Input: part model. Units: mm. Frame: model coordinates. A direction names the side the tool comes from. Round coordinates to 2 decimals unless told otherwise and drop trailing zeros. Loops run counter-clockwise (first coordinate to the right, second up) from the corner with the lowest first, then second, coordinate; pieces in that order, holes last.
1) Draft query along Z for faces 4 (the face through (-16, 2, 32.3)), 5 (the face through (-46, 2, -4)), 6 (the face through (-8, 2, -29)). Return one class per face: pulls with the +Z half, pulls with the -Z half, needs draft (parallel to the pull), parting line crosses it, or undercut.
2) Ray query, line 1 along X through (y, z) = (1.5, -10.5); line 2 along Z through (x, y) = (-41.5, 0.45). Return the intervals inside material, ascending.
3) Access query for faces 1 (the face through (-44, 2, -24)), 2 (the face through (44, 2, 25)), 3 (the face through (28, 2, 31)). Directions: +Z, -Z, +X, -X, +Y, -Y. A direction counts if a zero-diameter tool reaches every point of the face in a straight line with its end or side. Return the directions, or none.
4) First-contact query: pin 1 (1.6 mm diameter, centred on y = 1, z = 9, fed in from -X); pin 2 (1 mm diameter, centred on y = 1, z = -31.5, fed in from -X); pin 3 (1.5 mm diameter, centred on y = 3, z = 22, fed in from +X). Flat tips, straight axial feed; report the tip coordinate or a pass-through.
5) Section A-A, the plane x = -39. Return loops of the section in (y, z), and give its area (3 significant figures).
from build123d import *

# Parameters (mm, degrees)
ESQUISSE4_W                    = 88
ESQUISSE4_H                    = 58
BOSS_EXTRU_3_DEPTH             = 3.3
ESQUISSE5_W                    = 8
ESQUISSE5_H                    = 3.3
BOSS_EXTRU_6_DEPTH             = 3.3
R_P_TITION_LIN_AIRE2_COUNT     = 3
R_P_TITION_LIN_AIRE2_PITCH     = 16
R_P_TITION_LIN_AIRE2_COL_COUNT = 3
R_P_TITION_LIN_AIRE2_COL_PITCH = 16
SYM_TRIE1_COPY_1_SKETCH_W      = 8
SYM_TRIE1_COPY_1_SKETCH_H      = 3.3
SYM_TRIE1_COPY_1_DEPTH         = 3.3
SYM_TRIE1_COPY_2_SKETCH_W      = 8
SYM_TRIE1_COPY_2_SKETCH_H      = 3.3
SYM_TRIE1_COPY_2_DEPTH         = 3.3
SYM_TRIE1_COPY_3_SKETCH_W      = 8
SYM_TRIE1_COPY_3_SKETCH_H      = 3.3
SYM_TRIE1_COPY_3_DEPTH         = 3.3
SYM_TRIE1_COPY_4_SKETCH_W      = 8
SYM_TRIE1_COPY_4_SKETCH_H      = 3.3
SYM_TRIE1_COPY_4_DEPTH         = 3.3
ESQUISSE6_W                    = 3.3
ESQUISSE6_H                    = 8
BOSS_EXTRU_7_DEPTH             = 3.3
R_P_TITION_LIN_AIRE3_COUNT     = 2
R_P_TITION_LIN_AIRE3_PITCH     = 16
R_P_TITION_LIN_AIRE3_COL_COUNT = 2
R_P_TITION_LIN_AIRE3_COL_PITCH = 16
SYM_TRIE2_COPY_1_SKETCH_W      = 3.3
SYM_TRIE2_COPY_1_SKETCH_H      = 8
SYM_TRIE2_COPY_1_DEPTH         = 3.3
SYM_TRIE2_COPY_2_SKETCH_W      = 3.3
SYM_TRIE2_COPY_2_SKETCH_H      = 8
SYM_TRIE2_COPY_2_DEPTH         = 3.3


with BuildPart() as part:
    # Esquisse4 → Boss.-Extru.3 (new body)
    with BuildSketch(Plane(origin=(0, 0, 0), x_dir=(1, 0, 0), z_dir=(0, 1, 0))):
        Rectangle(ESQUISSE4_W, ESQUISSE4_H)
    extrude(amount=BOSS_EXTRU_3_DEPTH)

    # Esquisse5 → Boss.-Extru.6 (add)
    with BuildSketch(Plane.XZ):
        with Locations((0, 30.65)):
            Rectangle(ESQUISSE5_W, ESQUISSE5_H)
    boss_extru_6 = extrude(amount=-BOSS_EXTRU_6_DEPTH)

    # Répétition linéaire2: Boss.-Extru.6 ×3
    with Locations(*[(-i * R_P_TITION_LIN_AIRE2_PITCH, 0, 0) for i in range(1, R_P_TITION_LIN_AIRE2_COUNT)]):
        add(boss_extru_6)

    # Répétition linéaire2 col: Boss.-Extru.6 ×3
    with Locations(*[(i * R_P_TITION_LIN_AIRE2_COL_PITCH, 0, 0) for i in range(1, R_P_TITION_LIN_AIRE2_COL_COUNT)]):
        add(boss_extru_6)

    # Symétrie1: Boss.-Extru.6 across plane
    add(boss_extru_6.mirror(Plane.XY))

    # Symétrie1 copy 1 sketch → Symétrie1 copy 1 (add)
    with BuildSketch(Plane(origin=(-16, 0, 0), x_dir=(1, 0, 0), z_dir=(0, -1, 0))):
        with Locations((0, -30.65)):
            Rectangle(SYM_TRIE1_COPY_1_SKETCH_W, SYM_TRIE1_COPY_1_SKETCH_H)
    extrude(amount=-SYM_TRIE1_COPY_1_DEPTH)

    # Symétrie1 copy 2 sketch → Symétrie1 copy 2 (add)
    with BuildSketch(Plane(origin=(-32, 0, 0), x_dir=(1, 0, 0), z_dir=(0, -1, 0))):
        with Locations((0, -30.65)):
            Rectangle(SYM_TRIE1_COPY_2_SKETCH_W, SYM_TRIE1_COPY_2_SKETCH_H)
    extrude(amount=-SYM_TRIE1_COPY_2_DEPTH)

    # Symétrie1 copy 3 sketch → Symétrie1 copy 3 (add)
    with BuildSketch(Plane(origin=(16, 0, 0), x_dir=(1, 0, 0), z_dir=(0, -1, 0))):
        with Locations((0, -30.65)):
            Rectangle(SYM_TRIE1_COPY_3_SKETCH_W, SYM_TRIE1_COPY_3_SKETCH_H)
    extrude(amount=-SYM_TRIE1_COPY_3_DEPTH)

    # Symétrie1 copy 4 sketch → Symétrie1 copy 4 (add)
    with BuildSketch(Plane(origin=(32, 0, 0), x_dir=(1, 0, 0), z_dir=(0, -1, 0))):
        with Locations((0, -30.65)):
            Rectangle(SYM_TRIE1_COPY_4_SKETCH_W, SYM_TRIE1_COPY_4_SKETCH_H)
    extrude(amount=-SYM_TRIE1_COPY_4_DEPTH)

    # Esquisse6 → Boss.-Extru.7 (add)
    with BuildSketch(Plane.XZ):
        with Locations((-45.65, 0)):
            Rectangle(ESQUISSE6_W, ESQUISSE6_H)
    boss_extru_7 = extrude(amount=-BOSS_EXTRU_7_DEPTH)

    # Répétition linéaire3: Boss.-Extru.7 ×2
    with Locations(*[(0, 0, i * R_P_TITION_LIN_AIRE3_PITCH) for i in range(1, R_P_TITION_LIN_AIRE3_COUNT)]):
        add(boss_extru_7)

    # Répétition linéaire3 col: Boss.-Extru.7 ×2
    with Locations(*[(0, 0, -i * R_P_TITION_LIN_AIRE3_COL_PITCH) for i in range(1, R_P_TITION_LIN_AIRE3_COL_COUNT)]):
        add(boss_extru_7)

    # Symétrie2: Boss.-Extru.7 across plane
    add(boss_extru_7.mirror(Plane(origin=(0, 0, 0), x_dir=(0, 0, 1), z_dir=(1, 0, 0))))

    # Symétrie2 copy 1 sketch → Symétrie2 copy 1 (add)
    with BuildSketch(Plane(origin=(0, 0, 16), x_dir=(-1, 0, 0), z_dir=(0, -1, 0))):
        with Locations((-45.65, 0)):
            Rectangle(SYM_TRIE2_COPY_1_SKETCH_W, SYM_TRIE2_COPY_1_SKETCH_H)
    extrude(amount=-SYM_TRIE2_COPY_1_DEPTH)

    # Symétrie2 copy 2 sketch → Symétrie2 copy 2 (add)
    with BuildSketch(Plane(origin=(0, 0, -16), x_dir=(-1, 0, 0), z_dir=(0, -1, 0))):
        with Locations((-45.65, 0)):
            Rectangle(SYM_TRIE2_COPY_2_SKETCH_W, SYM_TRIE2_COPY_2_SKETCH_H)
    extrude(amount=-SYM_TRIE2_COPY_2_DEPTH)


solid = part.part
Final values:
1. face 4: pulls with the +Z half
1. face 5: undercut
1. face 6: pulls with the -Z half
2. line 1: x = -44 to 44
2. line 2: z = -29 to 29
3. face 1: -Z, -X, +Y, -Y
3. face 2: +Z, +X, +Y, -Y
3. face 3: +Z, +Y, -Y
4. pin 1: stops at x = -44
4. pin 2: stops at x = -36
4. pin 3: stops at x = 44
5. outline: (0, -29) - (3.3, -29) - (3.3, 29) - (0, 29) - close
5. area: 191 mm2
